Geometry: final body of the model. Coordinates: model frame, mm. Face numbers are marked on the shaded views. Give positions to 0.01 mm unless a question says otherwise; leave off trailing zeros. Order: outer loops, then holes, each group sorted by start corner. A loop starts at its lowest first (then second) coordinate and runs counter-clockwise, first axis right, second up. Notation, with made-up numbers: (-26, 7) - (28, 7) arc R31 cw to (28, 42) - close; hole circle Ø6 at (34.5, -9.5). An arc over 180 degrees is marked (long way). Write item = value, one per line. Start each with the question number.
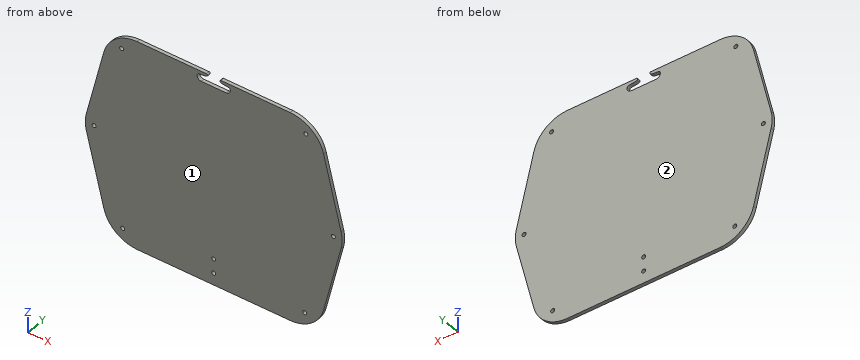
from build123d import *

# Parameters (mm, degrees)
EXTRUDE_1_DEPTH     = 3
SKETCH_2_R          = 1.75
CUT_EXTRUDE_1_DEPTH = 10
SKETCH_3_R          = 1.75
CUT_EXTRUDE_2_DEPTH = 10
SKETCH_4_R          = 1.75
CUT_EXTRUDE_3_DEPTH = 10
CUT_EXTRUDE_4_DEPTH = 10


with BuildPart() as part:
    # 草图1 → 凸台-拉伸1 (new body)
    with BuildSketch(Plane(origin=(0, 0, 0), x_dir=(1, 0, 0), z_dir=(0, 1, 0))):
        with BuildLine():
            Line((-66.78059141, 154.593992167), (66.78059141, 154.593992167))
            ThreePointArc((66.78059141, 154.593992167), (85.265515034, 148.222525736), (95.898700635, 131.814498742))
            Line((95.898700635, 131.814498742), (111.265547961, 69.844672358))
            ThreePointArc((111.265547961, 69.844672358), (112.147438737, 62.624165782), (111.265547961, 55.403659207))
            Line((111.265547961, 55.403659207), (95.898700635, -6.566167178))
            ThreePointArc((95.898700635, -6.566167178), (85.265515034, -22.974194171), (66.78059141, -29.345660602))
            Line((66.78059141, -29.345660602), (-66.78059141, -29.345660602))
            ThreePointArc((-66.78059141, -29.345660602), (-85.265515034, -22.974194171), (-95.898700635, -6.566167178))
            Line((-95.898700635, -6.566167178), (-111.265547961, 55.403659207))
            ThreePointArc((-111.265547961, 55.403659207), (-112.147438737, 62.624165782), (-111.265547961, 69.844672358))
            Line((-111.265547961, 69.844672358), (-95.898700635, 131.814498742))
            ThreePointArc((-95.898700635, 131.814498742), (-85.265515034, 148.222525736), (-66.78059141, 154.593992167))
        make_face()
    extrude(amount=EXTRUDE_1_DEPTH)

    # 草图2 → 切除-拉伸1 (cut)
    with BuildSketch(Plane(origin=(0, 3, 0), x_dir=(1, 0, 0), z_dir=(0, 1, 0))):
        with Locations(Location((-104.507530951, 62.624165782, 0), (0, 0, 270))):
            Circle(SKETCH_2_R)
        with Locations(Location((-80.450184708, -16.818951307, 0), (0, 0, 270))):
            Circle(SKETCH_2_R)
        with Locations(Location((104.507530951, 62.624165782, 0), (0, 0, 270))):
            Circle(SKETCH_2_R)
        with Locations(Location((80.450184708, -16.818951307, 0), (0, 0, 270))):
            Circle(SKETCH_2_R)
    extrude(amount=-CUT_EXTRUDE_1_DEPTH, mode=Mode.SUBTRACT)

    # 草图3 → 切除-拉伸2 (cut)
    with BuildSketch(Plane(origin=(0, 3, 0), x_dir=(1, 0, 0), z_dir=(0, 1, 0))):
        with Locations(Location((0, 131.568155221, 0), (0, 0, 270))):
            Circle(SKETCH_3_R)
        with Locations(Location((0, 144.079729864, 0), (0, 0, 270))):
            Circle(SKETCH_3_R)
    extrude(amount=-CUT_EXTRUDE_2_DEPTH, mode=Mode.SUBTRACT)

    # 草图4 → 切除-拉伸3 (cut)
    with BuildSketch(Plane(origin=(0, 3, 0), x_dir=(1, 0, 0), z_dir=(0, 1, 0))):
        with Locations(Location((-79.5, 141.78226533, 0), (0, 0, 270))):
            Circle(SKETCH_4_R)
        with Locations(Location((79.5, 141.78226533, 0), (0, 0, 270))):
            Circle(SKETCH_4_R)
    extrude(amount=-CUT_EXTRUDE_3_DEPTH, mode=Mode.SUBTRACT)

    # 草图5 → 切除-拉伸4 (cut)
    with BuildSketch(Plane(origin=(0, 3, 0), x_dir=(1, 0, 0), z_dir=(0, 1, 0))):
        with BuildLine():
            Line((11.016648097, -20.513898252), (-11.016648097, -20.513898252))
            ThreePointArc((-11.016648097, -20.513898252), (-13.814702514, -21.911306641), (-14.378457093, -24.987674549))
            add(Edge.make_bspline(
                [(-14.378457093, -24.987674549), (-14.050661547, -26.11933694), (-10.489346867, -26.76009099), (-7.724749574, -26.493757466), (-5.904508816, -27.417302496), (-5.804576355, -27.473305111)],
                knots=[0, 0, 0, 0, 0.274123853, 0.745489655, 0.777393608, 0.777393608, 0.777393608, 0.777393608], degree=3))
            ThreePointArc((-5.804576355, -27.473305111), (-5.325885634, -28.59829127), (-6.293448421, -29.345660602))
            Line((-6.293448421, -29.345660602), (6.293448421, -29.345660602))
            ThreePointArc((6.293448421, -29.345660602), (5.325885634, -28.59829127), (5.804576355, -27.473305111))
            add(Edge.make_bspline(
                [(5.804576355, -27.473305111), (5.904508816, -27.417302496), (7.724749574, -26.493757466), (10.489346867, -26.76009099), (14.050661547, -26.11933694), (14.378457093, -24.987674549)],
                knots=[0, 0, 0, 0, 0.031903952, 0.503269754, 0.777393608, 0.777393608, 0.777393608, 0.777393608], degree=3))
            ThreePointArc((14.378457093, -24.987674549), (13.814702514, -21.911306641), (11.016648097, -20.513898252))
        make_face()
    extrude(amount=-CUT_EXTRUDE_4_DEPTH, mode=Mode.SUBTRACT)


solid = part.part
Q1. Section B-B, the plane y = 0.6. Count the separate pieces of the cut face and the enclosed holes in it, then the cut area to 3 significant figures.
Q2. Material intervals for line 1 along X through (y, z) = (1.3, -63); line 2 along Z through (x, y) = (79, 2.3); line 3 along Z through (x, y) = (-1, 2.9), sorted ascending. Write a range as from..to.
Q3. Contact query for a flat-ended pin moving along its axis: pin 1 (3 mm diameter, centred on x = 104.51, z = -62.62, fed in from -Y). Output: stop coordinate, or through.
Q4. Section C-C, the plane z = -13.5. Return the cut outline in (x, y).
Q5. Pull-direction query (Y, two-part tool) for the marked faces 1 and 2; classes: +Y half, -Y half, draft (parallel to the pull), parting line (faces both ways), or undercut.
Q6. Section A-A, the plane z = -85.5. Return the cut outline in (x, y).
The answers:
q1.separate_pieces = 1
q1.enclosed_holes = 8
q1.area = 36,700 mm²
q2.line_1 = -112.15..-106.22, -102.8..102.8, 106.22..112.15
q2.line_2 = -151.99..-143.46, -140.11..15.84, 17.8..26.74
q2.line_3 = -154.59..-145.52, -142.64..-133, -130.13..20.51
q3.pin_1 = through
q4.outline = (-100.87, 0) - (100.87, 0) - (100.87, 3) - (-100.87, 3) - close
q5.face_1 = -Y half
q5.face_2 = +Y half
q6.outline = (-107.38, 0) - (107.38, 0) - (107.38, 3) - (-107.38, 3) - close
